```python
from build123d import *

# Parameters (mm, degrees)
SKETCH_R     = 0.65
PAD_DEPTH    = 10
POCKET_DEPTH = 10.001


with BuildPart() as part:
    # Sketch → Pad (new body)
    with BuildSketch(Plane.XY):
        with BuildLine():
            ThreePointArc((-32.05582, 12.757822), (-28.701718, 8.257822), (-25.347616, 12.757822))
            Line((-25.347616, 12.757822), (-26.305931, 15.972107))
            ThreePointArc((-26.305931, 15.972107), (-28.701718, 17.757822), (-31.097506, 15.972107))
            Line((-32.05582, 12.757822), (-31.097506, 15.972107))
        make_face()
        with Locations((-28.701718, 11.757822)):
            Circle(SKETCH_R, mode=Mode.SUBTRACT)
    extrude(amount=PAD_DEPTH)

    # Sketch001 (on Face7 of Pad) → Pocket (cut, through all)
    with BuildSketch(Plane.XY.offset(10)):
        with BuildLine():
            ThreePointArc((-30.785044, 13.316866), (-30.37172, 13.23769), (-29.951718, 13.211157))
            Line((-29.951718, 13.211157), (-27.451718, 13.211157))
            ThreePointArc((-27.451718, 13.211157), (-27.031717, 13.23769), (-26.618393, 13.316866))
            Line((-26.451718, 12.757822), (-26.618393, 13.316866))
            ThreePointArc((-26.451718, 12.757822), (-26.945875, 12.8726), (-27.451718, 12.911157))
            Line((-27.451718, 12.911157), (-29.951718, 12.911157))
            ThreePointArc((-29.951718, 12.911157), (-30.457562, 12.8726), (-30.951718, 12.757822))
            Line((-30.951718, 12.757822), (-30.785044, 13.316866))
        make_face()
    extrude(amount=-POCKET_DEPTH, mode=Mode.SUBTRACT)


solid = part.part
```
Design review of the part built by this model. Coordinates are the model's own, in mm. A direction names the side the tool comes from. Give positions to 0.01 mm unless a question says otherwise; leave off trailing zeros. Loops run counter-clockwise (first coordinate to the right, second up) from the corner with the lowest first, then second, coordinate; pieces in that order, holes last. Notation, with made-up numbers: (-2.75, 20.5) -> (24.25, 20.5) arc R14 cw to (24.25, 26.5) -> close; hole circle Ø5 at (59, 30.25). An arc over 180 degrees is marked (long way). Write each question's results on one line, items separated by ' | '.
Q1. Wall thickness on L1, parallel to Y at x = -28.5, z = 9.5; L2, parallel to Y at x = -28.25, z = 5; L3, parallel to Y at x = -30, z = 9.75: over which ranges is each line inside the solid? List them lowest first.
Reply:
L1: y = 8.26 to 11.14, 12.38 to 12.91, 13.21 to 17.75 | L2: y = 8.29 to 11.29, 12.23 to 12.91, 13.21 to 17.72 | L3: y = 8.51 to 12.91, 13.21 to 17.39
Q2. Take a section at C-C, the plane z = 8.75. Write out the cut boundary in (x, y).
Reply:
outline: (-32.06, 12.76) arc R3.5 ccw (long way) to (-25.35, 12.76) -> (-26.31, 15.97) arc R2.5 ccw to (-31.1, 15.97) -> close; hole (-30.95, 12.76) arc R3.34 cw to (-29.95, 12.91) -> (-27.45, 12.91) arc R3.34 cw to (-26.45, 12.76) -> (-26.62, 13.32) arc R3.34 cw to (-27.45, 13.21) -> (-29.95, 13.21) arc R3.34 cw to (-30.79, 13.32) -> close; hole circle Ø1.3 at (-28.7, 11.76)
Q3. Take a section at B-B, the plane x = -28.5. Write out the cut boundary in (y, z), plus the area to 3 significant figures.
Reply:
outline: (8.26, 0) -> (11.14, 0) -> (11.14, 10) -> (8.26, 10) -> close; (12.38, 0) -> (12.91, 0) -> (12.91, 10) -> (12.38, 10) -> close; (13.21, 0) -> (17.75, 0) -> (17.75, 10) -> (13.21, 10) -> close | area: 79.5 mm²
Q4. Take a section at D-D, the plane x = -27.75. Write out the cut boundary in (y, z), plus the area to 3 significant figures.
Reply:
outline: (8.39, 0) -> (12.91, 0) -> (12.91, 10) -> (8.39, 10) -> close; (13.21, 0) -> (17.57, 0) -> (17.57, 10) -> (13.21, 10) -> close | area: 88.8 mm²
Q5. The part is to be moulded in two halves that separate along X. For faces 3 (the face through (-29, 12.911, 5)), 4 (the face through (-26.94, 12.87, 5.07)), 5 (the face through (-31.583, 14.342, 4.93)), 6 (the face through (-28.79, 8.26, 4.93)), say which applies: +X half, -X half, draft (parallel to the pull), parting line (faces both ways), or undercut.
Reply:
face 3: undercut | face 4: undercut | face 5: -X half | face 6: parting line
Q6. Take a section at A-A, the plane x = -30.25. Write out the cut boundary in (y, z).
Reply:
outline: (8.62, 0) -> (12.9, 0) -> (12.9, 10) -> (8.62, 10) -> close; (13.22, 0) -> (17.22, 0) -> (17.22, 10) -> (13.22, 10) -> close
Q7. Machinability: for faces 1 (the face through (-30.38, 13.24, 5.07)), 2 (the face through (-25.82, 14.34, 4.93)), which of the approach directions +Z, -Z, +X, -X, +Y, -Y give a long, thin tool a straight path to every point of the face, cutting with its end or side? Answer none if there is none.
Reply:
face 1: +Z, -Z | face 2: +Z, -Z, +X, +Y
Q8. For pin 1 Ø1.5 at (x, y) = (-28.7, 11.76) entering from -Z; pin 2 Ø0.8 at (x, z) = (-28, 3.5) entering from -Y; pin 3 Ø2 at (y, z) = (10, 6) entering from +X, all flat-tipped, find the tip position at first contact; note any pin that passes through.
Reply:
pin 1: stops at z = 0 | pin 2: stops at y = 8.27 | pin 3: stops at x = -25.28
